Autodesk Inventor part; units mm, degrees
ref_plane "YZ Plane" through (0, 0, 0) normal (1, 0, 0) x (0, 1, 0)
ref_plane "XZ Plane" through (0, 0, 0) normal (0, 1, 0) x (-1, 0, 0)
ref_plane "XY Plane" through (0, 0, 0) normal (0, 0, 1) x (1, 0, 0)
sketch "スケッチ1" plane through (0, 0, 0) normal (0, 0, 1) x (1, 0, 0)
  circle A0 centre (0, 0) radius 1.5
  dimension "d0" = 3
extrude "押し出し1" add sketch "スケッチ1" along normal blind 25
sketch "スケッチ2" plane through (0, 0, 25) normal (0, 0, 1) x (1, 0, 0)
  circle A0 centre (0, 0) radius 1.5
  circle A1 centre (0, 0) radius 3
  dimension "d3" = 6
extrude "押し出し2" add sketch "スケッチ2" along normal blind 2 contours A0 | A1
fillet "フィレット1" radius 2 1 edges at (-3, 0, 27)
properties part number "M3ボタンボルト20" material "鋼、高強度、低合金"
The model under review builds one solid part; all positions refer to its coordinate system, in mm. A direction names the side the tool comes from. Round coordinates to 2 decimals unless told otherwise and drop trailing zeros. Loops run counter-clockwise (first coordinate to the right, second up) from the corner with the lowest first, then second, coordinate; pieces in that order, holes last. Notation, with made-up numbers: (80.5, 69.25) -> (89.5, 69.25) arc R19 cw to (89.5, 76.25) -> close; hole circle Ø5 at (85, -22.75). An arc over 180 degrees is marked (long way). One line per question, with ' | ' between items. Start each with the question number.
Item 1: For pin 1 (1.5 mm diameter, centred on x = 1.5, z = 14.5, fed in from -Y); pin 2 (1 mm diameter, centred on x = 1.5, z = 19.5, fed in from -Y), all flat-tipped, find the tip position at first contact; note any pin that passes through.
Item 2: Add section A-A, the plane z = 15.75. Write out the cut boundary in (x, y), then the cut area to 3 significant figures.
Item 3: Wall thickness on line 1 along Y through (x, z) = (0, 20); line 2 along X through (y, z) = (-0.25, 8.75); line 3 along Z through (x, y) = (0.75, 1): over which ranges is each line inside the solid? List them lowest first. Write a range as [from, to].
Item 4: Machinability: for faces 1 (the face through (0, 0, 0)), 2 (the face through (1.3, -1.3, 25)), which of the approach directions +Z, -Z, +X, -X, +Y, -Y give a long, thin tool a straight path to every point of the face, cutting with its end or side? Answer none if there is none.
Return value:
1) pin 1: stops at y = -1.3 | pin 2: stops at y = -1.12
2) outline: circle Ø3 at (0, 0) | area: 7.07 mm2
3) line 1: y = [-1.5, 1.5] | line 2: x = [-1.48, 1.48] | line 3: z = [0, 26.98]
4) face 1: -Z, +X, -X, +Y, -Y | face 2: -Z
